Geometry: final body of the model. Coordinates: model frame, mm. Face numbers are marked on the shaded views. A direction names the side the tool comes from. Round coordinates to 2 decimals unless told otherwise and drop trailing zeros. Write each loop counter-clockwise with the first axis right and the second up, starting at its lowest first coordinate (ties: lowest second). Pieces come first, ordered by that corner, then holes.
from build123d import *

# Parameters (mm, degrees)
ESBO_O1_W                            = 48
ESBO_O1_H                            = 120
RESSALTO_EXTRUS_O1_DEPTH             = 3
RESSALTO_EXTRUS_O2_DEPTH             = 28
ESBO_O3_W                            = 120
ESBO_O3_H                            = 48
RESSALTO_EXTRUS_O3_DEPTH             = 3
ESBO_O4_W                            = 5
ESBO_O4_H                            = 48
RESSALTO_EXTRUS_O4_DEPTH             = 47
ESBO_O5_R                            = 11
CORTE_EXTRUS_O1_DEPTH                = 5
ESBO_O6_R                            = 4.25
CORTE_EXTRUS_O2_DEPTH                = 110.489725545
FILETE1_R                            = 11
ESBO_O7_R                            = 6.75
CORTE_EXTRUS_O3_DEPTH                = 142.014183684
ESBO_O8_W                            = 20
ESBO_O8_H                            = 48
CORTE_EXTRUS_O4_DEPTH                = 80.906195004
ESBO_O12_R                           = 1.5
CORTE_EXTRUS_O5_DEPTH                = 3
ESCAREADO_PARA_SFHCS_M31_D           = 3.4
ESCAREADO_PARA_SFHCS_M31_DEPTH       = 3
ESCAREADO_PARA_SFHCS_M31_CSINK_D     = 6.72
ESCAREADO_PARA_SFHCS_M31_CSINK_ANGLE = 90
ESCAREADO_PARA_SFHCS_M31_TIP         = 1.021463052
ESBO_O18_R                           = 1.5
CORTE_EXTRUS_O6_DEPTH                = 5


with BuildPart() as part:
    # Esboço1 → Ressalto-extrusão1 (new body)
    with BuildSketch(Plane(origin=(0, 0, 0), x_dir=(0, 1, 0), z_dir=(0, 0, 1))):
        Rectangle(ESBO_O1_W, ESBO_O1_H)
    extrude(amount=RESSALTO_EXTRUS_O1_DEPTH)

    # Esboço2 → Ressalto-extrusão2 (add)
    with BuildSketch(Plane(origin=(0, 0, 0), x_dir=(1, 0, 0), z_dir=(0, 0, -1))):
        Polygon((-60, -20), (-60, -24), (60, -24), (60, 24), (-60, 24), (-60, 20), (56, 20), (56, -20), align=None)
    extrude(amount=RESSALTO_EXTRUS_O2_DEPTH)

    # Esboço3 → Ressalto-extrusão3 (add)
    with BuildSketch(Plane(origin=(0, 0, -28), x_dir=(1, 0, 0), z_dir=(0, 0, -1))):
        Rectangle(ESBO_O3_W, ESBO_O3_H)
    extrude(amount=RESSALTO_EXTRUS_O3_DEPTH)

    # Esboço4 → Ressalto-extrusão4 (add)
    with BuildSketch(Plane(origin=(0, 0, -31), x_dir=(1, 0, 0), z_dir=(0, 0, -1))):
        with Locations((-37.5, 0)):
            Rectangle(ESBO_O4_W, ESBO_O4_H)
        with Locations((57.5, 0)):
            Rectangle(ESBO_O4_W, ESBO_O4_H)
    extrude(amount=RESSALTO_EXTRUS_O4_DEPTH)

    # Esboço5 → Corte-extrusão1 (cut)
    with BuildSketch(Plane(origin=(-40, 0, 0), x_dir=(0, -1, 0), z_dir=(-1, 0, 0))):
        with Locations((0, -57)):
            Circle(ESBO_O5_R)
    extrude(amount=-CORTE_EXTRUS_O1_DEPTH, mode=Mode.SUBTRACT)

    # Esboço6 → Corte-extrusão2 (cut, through all)
    with BuildSketch(Plane.XZ.offset(24)):
        with Locations(Location((-15.5, -13.5, 0), (0, 0, 270))):
            Circle(ESBO_O6_R)
        with Locations(Location((35.5, -13.5, 0), (0, 0, 270))):
            Circle(ESBO_O6_R)
    extrude(amount=-CORTE_EXTRUS_O2_DEPTH, mode=Mode.SUBTRACT)

    # Filete1
    filete1_edges = [part.edges().sort_by_distance(p)[0] for p in [
        (-37.5, 24, -78),
        (-37.5, -24, -78),
        (57.5, -24, -78),
        (57.5, 24, -78),
    ]]
    fillet(filete1_edges, radius=FILETE1_R)

    # Esboço7 → Corte-extrusão3 (cut, through all)
    with BuildSketch(Plane(origin=(55, 0, 0), x_dir=(0, -1, 0), z_dir=(-1, 0, 0))):
        with Locations((0, -57)):
            Circle(ESBO_O7_R)
    extrude(amount=-CORTE_EXTRUS_O3_DEPTH, mode=Mode.SUBTRACT)

    # Esboço8 → Corte-extrusão4 (cut, through all)
    with BuildSketch(Plane(origin=(0, 0, -31), x_dir=(1, 0, 0), z_dir=(0, 0, -1))):
        with Locations((-50, 0)):
            Rectangle(ESBO_O8_W, ESBO_O8_H)
    extrude(amount=-CORTE_EXTRUS_O4_DEPTH, mode=Mode.SUBTRACT)

    # Esboço12 → Corte-extrusão5 (cut)
    with BuildSketch(Plane.XY.offset(3)):
        with Locations((-25, 0)):
            Circle(ESBO_O12_R)
    extrude(amount=-CORTE_EXTRUS_O5_DEPTH, mode=Mode.SUBTRACT)

    # Escareado para SFHCS M31
    with Locations(Plane(origin=(0, 0, 3), x_dir=(0, -1, 0), z_dir=(0, 0, 1))):
        with Locations((0, -25)):
            CounterSinkHole(ESCAREADO_PARA_SFHCS_M31_D / 2, ESCAREADO_PARA_SFHCS_M31_CSINK_D / 2, depth=ESCAREADO_PARA_SFHCS_M31_DEPTH, counter_sink_angle=ESCAREADO_PARA_SFHCS_M31_CSINK_ANGLE)
            with Locations((0, 0, -(ESCAREADO_PARA_SFHCS_M31_DEPTH + ESCAREADO_PARA_SFHCS_M31_TIP / 2))):  # 118° drill point
                Cone(0, ESCAREADO_PARA_SFHCS_M31_D / 2, ESCAREADO_PARA_SFHCS_M31_TIP, mode=Mode.SUBTRACT)

    # Esboço18 → Corte-extrusão6 (cut)
    with BuildSketch(Plane(origin=(-40, 0, 0), x_dir=(0, -1, 0), z_dir=(-1, 0, 0))):
        with Locations((-16, -33)):
            Circle(ESBO_O18_R)
        with Locations((16, -33)):
            Circle(ESBO_O18_R)
        with Locations((0, -73)):
            Circle(ESBO_O18_R)
    extrude(amount=-CORTE_EXTRUS_O6_DEPTH, mode=Mode.SUBTRACT)


solid = part.part
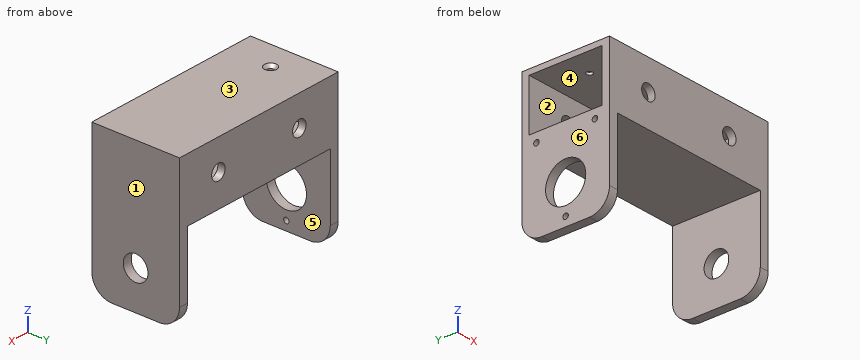
1) Section B-B on x = -32. Output: boundary loops of the cut face in (y, z).
2) Section A-A on y = 0. State how many separate pieces and enclosed holes the cut face has, plus the area to 3 significant figures.
3) Draft query along Z for the marked faces 1, 2 and 3. Return one class per face: pulls with the +Z half, pulls with the -Z half, needs draft (parallel to the pull), parting line crosses it, or undercut.
4) Reachability of the marked faces 4, 5 and 6 from +Z, -Z, +X, -X, +Y, -Y: full face, straight path, thin tool, end or side. Return the list, or none.
5) Line query: probe 1 along Z at (x, y) = (-36, 0); probe 2 along Y at (x, z) = (-18.5, -24.5); probe 3 along X at (y, z) = (12, -66). Output: solid intervals per line, ascending.
6) Section C-C on z = -33. Output: boundary loops of the cut face in (x, y), plus the area to 3 significant figures.
7) First-contact query: P1, Ø7, axis at x = 35.5, z = -13.5, coming from the -Y side; P2, Ø3, axis at y = -7.5, z = -6.5, coming from the -X side; P3, Ø14.5, axis at x = -8, y = -3, coming from the -Z side; P4, Ø2.5, axis at y = -16, z = -33, coming from the -X side. Flat tips, straight axial feed; report the tip coordinate or a pass-through.
8) Section D-D on x = 35.5. Output: boundary loops of the cut face in (y, z).
Filled in:
1. outline: (-24, -31) - (24, -31) - (24, 3) - (-24, 3) - close; hole (-20, -28) - (20, -28) - (20, 0) - (-20, 0) - close
2. separate pieces: 5
2. enclosed holes: 0
2. area: 977 mm2
3. face 1: needs draft
3. face 2: undercut
3. face 3: pulls with the +Z half
4. face 4: -X
4. face 5: -Z, +Y, -Y
4. face 6: +Z, -Z, -X, +Y, -Y
5. probe 1: z = -78 to -74.5, -71.5 to -68, -46 to -28, 0 to 3
5. probe 2: y = -24 to -20, 20 to 24
5. probe 3: x = -40 to -35, 55 to 60
6. outline: (-40, -24) - (-35, -24) - (-35, -17.5) - (-40, -17.5) - close; (-40, -14.5) - (-35, -14.5) - (-35, 14.5) - (-40, 14.5) - close; (-40, 17.5) - (-35, 17.5) - (-35, 24) - (-40, 24) - close; (55, -24) - (60, -24) - (60, 24) - (55, 24) - close
6. area: 450 mm2
7. P1: passes through
7. P2: stops at x = 56
7. P3: stops at z = -31
7. P4: stops at x = 55
8. outline: (-24, -31) - (24, -31) - (24, -17.75) - (20, -17.75) - (20, -28) - (-20, -28) - (-20, -17.75) - (-24, -17.75) - close; (-24, -9.25) - (-20, -9.25) - (-20, 0) - (20, 0) - (20, -9.25) - (24, -9.25) - (24, 3) - (-24, 3) - close
